from build123d import *

# Parameters (mm, degrees)
F1_DEPTH = 26
F2_DEPTH = 2
F3_R     = 0.6


with BuildPart() as f1:
    # F0 (on Top) → F1 (new body)
    with BuildSketch(Plane.XY):
        with BuildLine():
            ThreePointArc((-0.6565888179, -10.479450898), (-7.1887348474, 7.6532405747), (10.5, 0))
            ThreePointArc((10.5, 0), (7.6730926803, -7.1675413302), (0.7145431009, -10.4756588412))
            Line((0.7145431009, -10.4756588412), (0.7145431009, -11.5779716772))
            ThreePointArc((0.7145431009, -11.5779716772), (8.4512927996, -7.9457944861), (11.6, 0))
            ThreePointArc((11.6, 0), (-7.966918153, 8.431382754), (-0.6565888179, -11.5814028133))
            Line((-0.6565888179, -11.5814028133), (-0.6565888179, -10.479450898))
        make_face()
        with BuildLine():
            ThreePointArc((0.7145431009, -10.4756588412), (0.0290391056, -10.4999598442), (-0.6565888179, -10.479450898))
            Line((-0.6565888179, -10.479450898), (-0.6565888179, -11.5814028133))
            ThreePointArc((-0.6565888179, -11.5814028133), (0.0290278815, -11.5999636802), (0.7145431009, -11.5779716772))
            Line((0.7145431009, -11.5779716772), (0.7145431009, -10.4756588412))
        make_face()
    extrude(amount=F1_DEPTH)

    # F0 (on Top) → F2 (cut)
    with BuildSketch(Plane.XY):
        with BuildLine():
            ThreePointArc((0.7145431009, -10.4756588412), (0.0290391056, -10.4999598442), (-0.6565888179, -10.479450898))
            Line((-0.6565888179, -10.479450898), (-0.6565888179, -11.5814028133))
            ThreePointArc((-0.6565888179, -11.5814028133), (0.0290278815, -11.5999636802), (0.7145431009, -11.5779716772))
            Line((0.7145431009, -11.5779716772), (0.7145431009, -10.4756588412))
        make_face()
    extrude(amount=F2_DEPTH, mode=Mode.SUBTRACT)

    # F3
    f3_edges = [f1.edges().sort_by_distance(p)[0] for p in [
        (0.714543, -11.026815, 2),
        (-0.656589, -11.030427, 2),
    ]]
    fillet(f3_edges, radius=F3_R)


solid = f1.part
Can you work these out from the model? Positions are in its coordinate system, mm. A direction names the side the tool comes from. Give positions to 0.01 mm unless a question says otherwise; leave off trailing zeros. Loops run counter-clockwise (first coordinate to the right, second up) from the corner with the lowest first, then second, coordinate; pieces in that order, holes last. Notation, with made-up numbers: (-8, 52.5) - (27, 52.5) arc R20 cw to (27, 83.5) - close; hole circle Ø8 at (85.25, 56). An arc over 180 degrees is marked (long way). Return JSON: item names as keys, results as strings.
1. We'd pull the mould along X, two halves only. Please class faces 1 (the face through (-0.657, -11, 1)), 2 (the face through (-6, 9, 26)): +X half, -X half, draft (parallel to the pull), parting line (faces both ways), or undercut.
Output values:
{"face 1": "undercut", "face 2": "draft"}
2. I want a section at B-B on x = -8.25. Please give me the cut outline in (y, z).
Output values:
{"outline": "(-8.15, 0) - (-6.5, 0) - (-6.5, 26) - (-8.15, 26) - close; (6.5, 0) - (8.15, 0) - (8.15, 26) - (6.5, 26) - close"}
3. For faces 3 (the face through (5.1, -9.4, 0)), 4 (the face through (0.715, -11, 1)), which set-ups out of +Z, -Z, +X, -X, +Y, -Y let a thin tool reach every point of the face, with its end or its side?
Output values:
{"face 3": "-Z, +X, -X, +Y, -Y", "face 4": "-Z, -Y"}
4. If I drill on line 1 (Y direction, x = 0, z = 23); line 2 (Y direction, x = 2.75, z = 12.25), over which ranges is the centre line in solid material (lowest first)?
Output values:
{"line 1": "y = -11.6 to -10.5, 10.5 to 11.6", "line 2": "y = -11.27 to -10.13, 10.13 to 11.27"}
5. I want a section at A-A on y = 10. Please give me the cut outline in (x, z).
Output values:
{"outline": "(-5.88, 0) - (-3.2, 0) - (-3.2, 26) - (-5.88, 26) - close; (3.2, 0) - (5.88, 0) - (5.88, 26) - (3.2, 26) - close"}
6. I want a section at C-C on z = 12.5. Please give me the cut outline in (x, y).
Output values:
{"outline": "circle Ø23.2 at (0, 0); hole circle Ø21 at (0, 0)"}
7. I'm going to push flat-ended pins straight in: pin 1 Ø1 at (y, z) = (9, 12) entering from -X; pin 2 Ø4 at (y, z) = (-8.5, 16) entering from +X; pin 3 Ø5 at (x, y) = (-5.5, -2) entering from -Z; pin 4 Ø4 at (x, z) = (4, 12.5) entering from -Y. Where does each tip first touch, or does it pass through?
Output values:
{"pin 1": "stops at x = -7.89", "pin 2": "stops at x = 9.61", "pin 3": "passes through", "pin 4": "stops at y = -11.43"}
